from build123d import *

# Parameters (mm, degrees)
SKETCH_2_R          = 1.5
EXTRUDE_1_DEPTH     = 22
CUT_EXTRUDE_1_DEPTH = 1.04
CHAMFER_1_SIZE      = 0.2


with BuildPart() as part:
    # 草图1 → 旋转1 (revolve)
    with BuildSketch(Plane.XY, mode=Mode.PRIVATE) as revolve_1_sk:
        with BuildLine():
            Line((0, 0), (-2.775, 0))
            ThreePointArc((-2.775, 0), (-2.662639591, 0.78164916), (-2.334657362, 1.5))
            Line((-2.334657362, 1.5), (0, 1.5))
            Line((0, 1.5), (0, 0))
        make_face()
    revolve(revolve_1_sk.sketch.rotate(Axis((0, 5.111773046, 0), (0, -1, 0)), 270), axis=Axis((0, 5.111773046, 0), (0, -1, 0)))

    # 草图2 → 凸台-拉伸1 (add)
    with BuildSketch(Plane.XZ):
        with Locations(Location((0, 0, 0), (0, 0, 270))):
            Circle(SKETCH_2_R)
    extrude(amount=EXTRUDE_1_DEPTH)

    # 草图3 → 切除-拉伸1 (cut)
    with BuildSketch(Plane(origin=(0, 1.5, 0), x_dir=(1, 0, 0), z_dir=(0, 1, 0))):
        Polygon((0, 1.172021046), (-1.015, 0.586010523), (-1.015, -0.586010523), (0, -1.172021046), (1.015, -0.586010523), (1.015, 0.586010523), align=None)
    extrude(amount=-CUT_EXTRUDE_1_DEPTH, mode=Mode.SUBTRACT)

    # 倒角1
    chamfer_1_edges = [part.edges().sort_by_distance(p)[0] for p in [
        (0, -22, 1.5),
    ]]
    chamfer(chamfer_1_edges, length=CHAMFER_1_SIZE)


solid = part.part
The model under review builds one solid part; all positions refer to its coordinate system, in mm. A direction names the side the tool comes from. Coordinates: 2 decimals unless noted, no trailing zeros. Write each loop counter-clockwise with the first axis right and the second up, starting at its lowest first coordinate (ties: lowest second). Pieces come first, ordered by that corner, then holes. Notation, with made-up numbers: M 87,-29.5 L 96,-29.5 A15 ccw 96,-15.5 Z; hole C 82,62.25 d11. An arc over 180 degrees is marked long. Put each result on its own line as item: value.
1) For faces 1 (the flat face through (1.2, 0, -1.2)), 2 (the flat face through (0, -22, 0)), 3 (the flat face through (1.015, 1, 0)), list the 3-axis set-ups (+Z, -Z, +X, -X, +Y, -Y) from which the entire face can be reached by the end or side of a thin tool; tool diameter is ignored.
Computed:
face 1: -Y
face 2: +Z, -Z, +X, -X, -Y
face 3: +Y
2) Draft analysis for pull direction Z (two halves, no side actions). For faces 4 (the flat face through (-0.5, 0.987, -0.883)), 5 (the flat face through (-1, 1.5, 1)), 6 (the cylindrical face through (0.45, -10.75, -1.43)), state which applies: released by +Z, released by -Z, zero draft, split by the parting line, or undercut.
Computed:
face 4: undercut
face 5: zero draft
face 6: split by the parting line
3) Wall thickness on probe 1 along Y at (x, z) = (-2.15, 0.1); probe 2 along Z at (x, y) = (0.75, -16.5); probe 3 along Y at (x, z) = (-2.3, 0.75): over which ranges is each line inside the solid? List them lowest first. Write a range as [from, to].
Computed:
probe 1: y = [0, 1.5]
probe 2: z = [-1.3, 1.3]
probe 3: y = [0, 1.36]
4) Add section D-D on z = -1.85. Give the boundary of the cut face in (x, y).
Computed:
outline: M -2.07,0 L 2.07,0 A2.07 ccw 1.42,1.5 L -1.42,1.5 A2.07 ccw Z
5) Clearance check with flat-ended pins moving along their axes: pin 1 Ø1 at (y, z) = (-14.5, -0.5) entering from +X; pin 2 Ø1 at (x, z) = (-0.5, 0.5) entering from +Y; pin 3 Ø1.5 at (y, z) = (-7, -1.5) entering from -X; pin 4 Ø1.1 at (y, z) = (1, 0.5) entering from -X. State where each tip first meets the part, or that it passes through.
Computed:
pin 1: stops at x = 1.5
pin 2: stops at y = 1.5
pin 3: stops at x = -1.3
pin 4: stops at x = -2.72
6) Add section B-B on y = -3.75. Give the boundary of the cut face in (x, z), then the cut area to 3 significant figures.
Computed:
outline: C 0,0 d3
area: 7.07 mm2
7) Add section A-A on z = 0. Give the boundary of the cut face in (x, y) (3 decimals), then the cut area to 3 significant figures.
Computed:
outline: M -2.775,0 L -1.5,0 L -1.5,-21.8 L -1.3,-22 L 1.3,-22 L 1.5,-21.8 L 1.5,0 L 2.775,0 A2.775 ccw 2.335,1.5 L 1.015,1.5 L 1.015,0.46 L -1.015,0.46 L -1.015,1.5 L -2.335,1.5 A2.775 ccw Z
area: 71.7 mm2
8) Add section C-C on x = -2.05. Give the boundary of the cut face in (y, z), then the cut area to 3 significant figures.
Computed:
outline: M 0,-1.87 A1.87 ccw 1.5,-1.12 L 1.5,1.12 A1.87 ccw 0,1.87 Z
area: 4.93 mm2
